Work out the finished part from the listing and answer in its coordinate system (mm). A direction names the side the tool comes from. Coordinates: 2 decimals unless noted, no trailing zeros. Order: outer loops, then holes, each group sorted by start corner. A loop starts at its lowest first (then second) coordinate and runs counter-clockwise, first axis right, second up. Notation, with made-up numbers: M -35.5,44.5 L -11.5,44.5 A15 ccw -11.5,55.5 Z; hole C 79.5,49.5 d7. An arc over 180 degrees is marked long. Use a Markdown table: item, result.
from build123d import *

# Parameters (mm, degrees)
SKETCH1_R           = 16
SKETCH1_R_2         = 11.4
BOSS_EXTRUDE1_DEPTH = 6.7
SKETCH2_R           = 16
SKETCH2_R_2         = 10.7
BOSS_EXTRUDE2_DEPTH = 3.2
SKETCH3_R           = 16
SKETCH3_R_2         = 6.2
BOSS_EXTRUDE3_DEPTH = 1
SKETCH4_R           = 16
SKETCH4_R_2         = 4.7
BOSS_EXTRUDE4_DEPTH = 7
SKETCH5_R           = 16
SKETCH5_R_2         = 3
BOSS_EXTRUDE5_DEPTH = 7.5
SKETCH6_R           = 1.7
CUT_EXTRUDE1_DEPTH  = 25.4


with BuildPart() as part:
    # Sketch1 → Boss-Extrude1 (new body)
    with BuildSketch(Plane(origin=(0, 0, 0), x_dir=(0, 0, -1), z_dir=(1, 0, 0))):
        Circle(SKETCH1_R)
        Circle(SKETCH1_R_2, mode=Mode.SUBTRACT)
    extrude(amount=BOSS_EXTRUDE1_DEPTH)

    # Sketch2 → Boss-Extrude2 (add)
    with BuildSketch(Plane(origin=(6.7, 0, 0), x_dir=(0, 0, -1), z_dir=(1, 0, 0))):
        Circle(SKETCH2_R)
        Circle(SKETCH2_R_2, mode=Mode.SUBTRACT)
    extrude(amount=BOSS_EXTRUDE2_DEPTH)

    # Sketch3 → Boss-Extrude3 (add)
    with BuildSketch(Plane(origin=(9.9, 0, 0), x_dir=(0, 0, -1), z_dir=(1, 0, 0))):
        Circle(SKETCH3_R)
        Circle(SKETCH3_R_2, mode=Mode.SUBTRACT)
    extrude(amount=BOSS_EXTRUDE3_DEPTH)

    # Sketch4 → Boss-Extrude4 (add)
    with BuildSketch(Plane(origin=(10.9, 0, 0), x_dir=(0, 0, -1), z_dir=(1, 0, 0))):
        Circle(SKETCH4_R)
        Circle(SKETCH4_R_2, mode=Mode.SUBTRACT)
    extrude(amount=BOSS_EXTRUDE4_DEPTH)

    # Sketch5 → Boss-Extrude5 (add)
    with BuildSketch(Plane(origin=(17.9, 0, 0), x_dir=(0, 0, -1), z_dir=(1, 0, 0))):
        Circle(SKETCH5_R)
        with Locations(Location((0, 0, 0), (0, 0, 180))):
            Circle(SKETCH5_R_2, mode=Mode.SUBTRACT)
    extrude(amount=BOSS_EXTRUDE5_DEPTH)

    # Sketch6 → Cut-Extrude1 (cut)
    with BuildSketch(Plane(origin=(25.4, 0, 0), x_dir=(0, 0, -1), z_dir=(1, 0, 0))):
        with Locations((0, 8)):
            Circle(SKETCH6_R)
        with Locations((0, -8)):
            Circle(SKETCH6_R)
    extrude(amount=-CUT_EXTRUDE1_DEPTH, mode=Mode.SUBTRACT)


solid = part.part
(1) A cutting plane is placed at A-A (y = 0). Determine the outline of the cut face in (x, z), then the cut area to 3 significant figures.
Conclusion:
| item | result |
|---|---|
| outline | M 0,-16 L 25.4,-16 L 25.4,-3 L 17.9,-3 L 17.9,-4.7 L 10.9,-4.7 L 10.9,-6.2 L 9.9,-6.2 L 9.9,-10.7 L 6.7,-10.7 L 6.7,-11.4 L 0,-11.4 Z; M 0,11.4 L 6.7,11.4 L 6.7,10.7 L 9.9,10.7 L 9.9,6.2 L 10.9,6.2 L 10.9,4.7 L 17.9,4.7 L 17.9,3 L 25.4,3 L 25.4,16 L 0,16 Z |
| area | 468 mm2 |
(2) Determine the mould class of faces 3 (the flat face through (25.4, 0.2, -3.3)), 4 (the flat face through (9.9, -5, -5)), 5 (the cylindrical face through (12.52, -15.62, 3.47)) for opening direction Y: pulls with the +Y half, pulls with the -Y half, needs draft (parallel to the pull), parting line crosses it, or undercut.
Conclusion:
| item | result |
|---|---|
| face 3 | needs draft |
| face 4 | undercut |
| face 5 | parting line crosses it |
(3) Which of the six approach directions +Z, -Z, +X, -X, +Y, -Y give full straight-line access (tool end or side, diameter ignored) to faces 1 (the flat face through (10.9, 5, 1)), 2 (the cylindrical face through (21.6, -0.9, 2.86))?
Conclusion:
| item | result |
|---|---|
| face 1 | -X |
| face 2 | +X, -X |
(4) Given P1, Ø11.5, axis at y = 2.5, z = 5, coming from the -X side; P2, Ø8, axis at x = 8, z = -8.5, coming from the +Y side; P3, Ø6.5, axis at y = -2, z = -4, coming from the -X side, each flat-ended and moving along its own axis, determine where each tip first touches the part or whether it passes through.
Conclusion:
| item | result |
|---|---|
| P1 | x = 6.7 |
| P2 | y = 15.35 |
| P3 | x = 9.9 |
(5) A cutting plane is placed at C-C (z = -3.5). Determine the outline of the cut face in (x, y), then the cut area to 3 significant figures.
Conclusion:
| item | result |
|---|---|
| outline | M 0,-15.61 L 25.4,-15.61 L 25.4,15.61 L 0,15.61 L 0,10.85 L 6.7,10.85 L 6.7,10.11 L 9.9,10.11 L 9.9,5.12 L 10.9,5.12 L 10.9,3.14 L 17.9,3.14 L 17.9,-3.14 L 10.9,-3.14 L 10.9,-5.12 L 9.9,-5.12 L 9.9,-10.11 L 6.7,-10.11 L 6.7,-10.85 L 0,-10.85 Z |
| area | 529 mm2 |
(6) Straight lines are drawn through the part: L1, parallel to Y at x = 23.75, z = 0; L2, parallel to Y at x = 8.6, z = 0; L3, parallel to X at y = 6, z = -2. For each, find the intervals that lie inside material, in ascending order.
Conclusion:
| item | result |
|---|---|
| L1 | -16 to -9.7, -6.3 to -3, 3 to 6.3, 9.7 to 16 |
| L2 | -16 to -10.7, 10.7 to 16 |
| L3 | 9.9 to 25.4 |
(7) A cutting plane is placed at D-D (x = 1.5). Determine the outline of the cut face in (y, z), then the cut area to 3 significant figures.
Conclusion:
| item | result |
|---|---|
| outline | C 0,0 d32; hole C 0,0 d22.8 |
| area | 396 mm2 |
(8) A cutting plane is placed at B-B (x = 13.5). Determine the outline of the cut face in (y, z), then the cut area to 3 significant figures.
Conclusion:
| item | result |
|---|---|
| outline | C 0,0 d32; hole C -8,0 d3.4; hole C 0,0 d9.4; hole C 8,0 d3.4 |
| area | 717 mm2 |
